Design review of the part built by this model. Coordinates are the model's own, in mm. Coordinates: 2 decimals unless noted, no trailing zeros. Write each loop counter-clockwise with the first axis right and the second up, starting at its lowest first coordinate (ties: lowest second). Pieces come first, ordered by that corner, then holes. Notation, with made-up numbers: (-3.5, -8.75) - (16.5, -8.75) arc R23 ccw to (16.5, -0.75) - close; hole circle Ø7 at (62, -3.5). An arc over 180 degrees is marked (long way). One line per item, written item: value.
Autodesk Inventor part; units mm, degrees
ref_plane "YZ Plane" through (0, 0, 0) normal (1, 0, 0) x (0, 1, 0)
ref_plane "XZ Plane" through (0, 0, 0) normal (0, 1, 0) x (-1, 0, 0)
ref_plane "XY Plane" through (0, 0, 0) normal (0, 0, 1) x (1, 0, 0)
sketch "Sketch1" plane through (0, 0, 0) normal (0, 1, 0) x (-1, 0, 0)
  circle A0 centre (0, 0) radius 15.75
  circle A1 centre (0, 0) radius 25
  dimension "d0" = 31.5
  dimension "d1" = 50
extrude "Extrusion1" add sketch "Sketch1" along normal blind 70
sketch "Sketch2" plane through (0, 0, 0) normal (0, -1, 0) x (1, 0, 0)
  circle A0 centre (0, 0) radius 25
  circle A1 centre (0, 0) radius 30
  dimension "d4" = 5
extrude "Extrusion2" add sketch "Sketch2" against normal blind 3
fillet "Fillet1" radius 1 1 edges at (-30, 3, 0)
fillet "Fillet2" radius 3 2 edges at (15.75, 70, 0) (25, 70, 0)
properties part number "Adaptador rollo 5cm"
1. Consider section C-C, the plane y = 39. Write out the cut boundary in (x, z), then the cut area to 3 significant figures.
Answer block:
outline: circle Ø50 at (0, 0); hole circle Ø31.5 at (0, 0)
area: 1,180 mm^2
2. Consider section A-A, the plane x = 0. Write out the cut boundary in (y, z), then the cut area to 3 significant figures.
Answer block:
outline: (0, -30) - (2, -30) arc R1 ccw to (3, -29) - (3, -25) - (67, -25) arc R3 ccw to (70, -22) - (70, -18.75) arc R3 ccw to (67, -15.75) - (0, -15.75) - close; (0, 15.75) - (67, 15.75) arc R3 ccw to (70, 18.75) - (70, 22) arc R3 ccw to (67, 25) - (3, 25) - (3, 29) arc R1 ccw to (2, 30) - (0, 30) - close
area: 1,320 mm^2
3. Consider section B-B, the plane z = 0. Write out the cut boundary in (x, y).
Answer block:
outline: (-30, 0) - (-15.75, 0) - (-15.75, 67) arc R3 ccw to (-18.75, 70) - (-22, 70) arc R3 ccw to (-25, 67) - (-25, 3) - (-29, 3) arc R1 ccw to (-30, 2) - close; (15.75, 0) - (30, 0) - (30, 2) arc R1 ccw to (29, 3) - (25, 3) - (25, 67) arc R3 ccw to (22, 70) - (18.75, 70) arc R3 ccw to (15.75, 67) - close
4. Wall thickness on line 1 along Z through (x, y) = (0, 23); line 2 along X through (y, z) = (7.5, 7.5); line 3 along Z through (x, y) = (5.5, 8): over which ranges is each line inside the solid? List them lowest first.
Answer block:
line 1: z = -25 to -15.75, 15.75 to 25
line 2: x = -23.85 to -13.85, 13.85 to 23.85
line 3: z = -24.39 to -14.76, 14.76 to 24.39
5. Mouldability with a two-part tool opening along Z and no side actions: class faces 1 (the face through (13, 3, 22)), 2 (the face through (-23.846, 34.552, -7.509)), 3 (the face through (2.05, 33.031, -15.616)) as released by +Z, released by -Z, zero draft, split by the parting line, or undercut.
Answer block:
face 1: zero draft
face 2: split by the parting line
face 3: undercut
6. Insertion check: pin 1 Ø2 at (y, z) = (44.5, -20.5) entering from +X; pin 2 Ø5 at (y, z) = (58.5, 21.5) entering from +X; pin 3 Ø6 at (y, z) = (9.5, -17) entering from -X; pin 4 Ø25 at (x, z) = (0, 0) entering from -Y. Each pin has a flat end and moves straight along its axis. Give the tip position at first contact, or say it passes through.
Answer block:
pin 1: stops at x = 15.64
pin 2: stops at x = 16.25
pin 3: stops at x = -20.71
pin 4: passes through
